Design review of the part built by this model. Coordinates are the model's own, in mm. A direction names the side the tool comes from. Give positions to 0.01 mm unless a question says otherwise; leave off trailing zeros. Write each loop counter-clockwise with the first axis right and the second up, starting at its lowest first coordinate (ties: lowest second). Pieces come first, ordered by that corner, then holes.
```python
from build123d import *

# Parameters (mm, degrees)
F0_W          = 5.08
F0_H          = 5.08
F2_DEPTH      = 2.54
F2_DEPTH_BACK = 2.54
F3_SIZE2      = 2.53999
F3_SIZE       = 2.53999


# Not quite as in the source:
# - a fillet or chamfer is up to 0.001 mm smaller than in the source, because OpenCascade refuses the exact size


with BuildPart() as f1:
    # F0 (on Front) → F1 (revolve)
    with BuildSketch(Plane.XZ):
        with BuildLine():
            Line((-120.65, 0), (-19.05, 0))
            Line((-19.05, 0), (-19.05, 2.54))
            Line((-19.05, 2.54), (-19.05, 3.81))
            ThreePointArc((-19.05, 3.81), (-25.8165229562, 14.8770320486), (-38.1, 19.0461114431))
            Line((-38.1, 19.0461114431), (-38.1, 30.2734401025))
            Line((-38.1, 30.2734401025), (-50.8, 19.0461114431))
            Line((-50.8, 19.0461114431), (-50.8, 23.4911114431))
            Line((-50.8, 23.4911114431), (-55.88, 19.0461114431))
            Line((-55.88, 19.0461114431), (-62.23, 19.0461114431))
            Line((-62.23, 19.0461114431), (-62.23, 23.4911114431))
            Line((-62.23, 23.4911114431), (-66.675, 19.0461114431))
            ThreePointArc((-66.675, 19.0461114431), (-85.4281931482, 19.6893537461), (-101.6, 29.2061114431))
            Line((-101.6, 29.2061114431), (-101.6, 36.83))
            Line((-101.6, 36.83), (-110.49, 36.83))
            Line((-110.49, 36.83), (-110.49, 44.45))
            Line((-110.49, 44.45), (-120.65, 44.45))
            Line((-120.65, 44.45), (-120.65, 0))
        make_face()
    revolve(axis=Axis((-69.85, 0, 0), (-1, 0, 0)))

    # F0 (on Front) → F2 (join, two sides)
    with BuildSketch(Plane.XZ) as f2_sk:
        with Locations((-2.54, 0)):
            Rectangle(F0_W, F0_H)
        with Locations((-7.62, -5.08)):
            Rectangle(F0_W, F0_H)
        with Locations((-7.62, 0)):
            Rectangle(F0_W, F0_H)
        with Locations((-7.62, 5.08)):
            Rectangle(F0_W, F0_H)
        Polygon((-19.05, 2.54), (-19.05, 0), (-19.05, -2.54), (-10.16, -2.54), (-10.16, 2.54), align=None)
    extrude(amount=F2_DEPTH)
    extrude(f2_sk.sketch, amount=-F2_DEPTH_BACK)

    # F3 (size 2.54 and 2.54 in the source; OpenCascade refuses exactly that, so slightly less here)
    f3_edges = [f1.edges().sort_by_distance(p)[0] for p in [
        (-10.16, 0, 7.62),
        (-5.08, 0, 7.62),
        (0, 0, 2.54),
        (0, 0, -2.54),
        (-5.08, 0, -7.62),
        (-10.16, 0, -7.62),
    ]]
    chamfer(f3_edges, length=F3_SIZE, length2=F3_SIZE2)


solid = f1.part
```
(1) Consider section A-A, the plane x = -58.5. Give the boundary of the cut face in (y, z), then the cut area to 3 significant figures.
Resolved:
outline: circle Ø38.09 at (0, 0)
area: 1,140 mm2
(2) Consider section B-B, the plane z = -39. Give the boundary of the cut face in (x, y), then the cut area to 3 significant figures.
Resolved:
outline: (-120.65, -21.33) - (-110.49, -21.33) - (-110.49, 21.33) - (-120.65, 21.33) - close
area: 433 mm2
(3) Tool access review of faces 5 (the face through (-19.05, 0, 3)), 6 (the face through (-110.49, 33, 17)), 7 (the face through (-10, 2.54, 0)): name each direction out of +Z, -Z, +X, -X, +Y, -Y from which nothing blocks a thin tool from reaching the whole face with its end or side.
Resolved:
face 5: none
face 6: +X
face 7: +Z, -Z, +X, +Y
(4) To check wall thickness, follow L1, parallel to Y at x = -102.5, z = 21; L2, parallel to Y at x = -17.5, z = 2; L3, parallel to X at y = -20.5, z = 32.5. State the ranges of each line that lie inside material, in increasing order.
Resolved:
L1: y = -30.26 to 30.26
L2: y = -2.54 to 2.54
L3: x = -120.65 to -110.49
(5) Clearance check with flat-ended pins moving along their axes: P1, Ø5.5, axis at x = -15, y = 0.5, coming from the -Z side; P2, Ø14, axis at y = 10.5, z = 8.5, coming from the +X side; P3, Ø3, axis at y = 0.5, z = 3.5, coming from the +X side. State where each tip first meets the part, or that it passes through.
Resolved:
P1: stops at z = -2.54
P2: stops at x = -19.81
P3: stops at x = -2
(6) Mouldability with a two-part tool opening along X and no side actions: class faces 1 (the face through (-15, 0, 2.54)), 2 (the face through (-38.1, -20, 0)), 3 (the face through (-120.65, 1, -1)), 4 (the face through (-15, 0, -2.54)) as pulls with the +X half, pulls with the -X half, needs draft (parallel to the pull), parting line crosses it, or undercut.
Resolved:
face 1: undercut
face 2: pulls with the +X half
face 3: pulls with the -X half
face 4: undercut
(7) Consider section D-D, the plane x = -40. Give the boundary of the cut face in (y, z).
Resolved:
outline: circle Ø57.19 at (0, 0)
